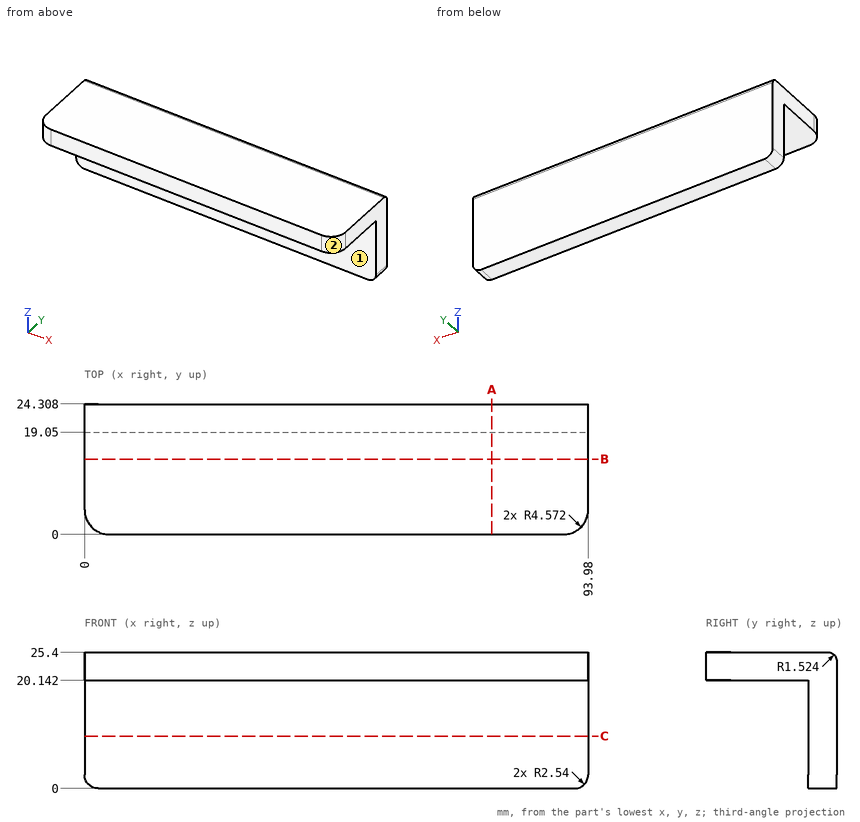
Here's the drawing with two shaded views (mm, measured from the low corner). I have some questions. A direction names the side the tool comes from. Coordinates: 2 decimals unless noted, no trailing zeros. Write each loop counter-clockwise with the first axis right and the second up, starting at its lowest first coordinate (ties: lowest second). Pieces come first, ordered by that corner, then holes. Notation, with made-up numbers: (-11, 59.25) -> (34, 59.25) arc R27 cw to (34, 80.25) -> close; hole circle Ø8 at (1.5, 29). An arc over 180 degrees is marked (long way). Answer as CSV lines item,"result".
1) If we section it at C-C on z = 9.75: Please give me the cut outline in (x, y), then the cut area to 3 significant figures.
Check result:
outline,"(0, 19.05) -> (93.98, 19.05) -> (93.98, 24.31) -> (0, 24.31) -> close"
area,"494 mm²"
2) On a 3-axis mill with a long thin cutter (end or side, diameter ignored), from which of +Z, -Z, +X, -X, +Y, -Y can I reach the whole of each face in a straight line? I mean the marked faces 1 and 2. Say none if no direction works.
Check result:
face 1,"-Z, +X, -X, -Y"
face 2,"+Z, -Z, +X, -Y"
3) If I drill on line 1 (Z direction, x = 78.5, y = 4.5); line 2 (Y direction, x = 20.5, z = 11.5), over which ranges is the centre line in solid material (lowest first)? Write a range as from..to.
Check result:
line 1,"20.14..25.4"
line 2,"19.05..24.31"
4) If we section it at A-A on x = 76: Please give me the cut outline in (y, z).
Check result:
outline,"(0, 20.14) -> (19.05, 20.14) -> (19.05, 0) -> (24.31, 0) -> (24.31, 23.88) arc R1.52 ccw to (22.78, 25.4) -> (0, 25.4) -> close"
5) If we section it at B-B on y = 14: Please give me the cut outline in (x, z).
Check result:
outline,"(0, 20.14) -> (93.98, 20.14) -> (93.98, 25.4) -> (0, 25.4) -> close"
